from build123d import *

# Parameters (mm, degrees)
BASE_DEPTH                     = 3
CONG_1_R                       = 3
ESQUISSE20_R                   = 3
PER_AGE_PROFIL_S_DEPTH         = 4
ESQUISSE21_R                   = 1.65
PER_AGE_LIDAR_DEPTH            = 4
ESQUISSE22_R                   = 11.25
PER_AGE_ARRET_D_URGENCE_DEPTH  = 4
ESQUISSE23_R                   = 7
PER_AGE_TIRETTE_DEPTH          = 4
ESQUISSE24_W                   = 68
ESQUISSE24_H                   = 207
PER_AGE_CABLE_MANAGEMENT_DEPTH = 4


with BuildPart() as part:
    # Esquisse1 → Base (new body)
    with BuildSketch(Plane.XY):
        Polygon((0, 0), (-200, 0), (-224.748737342, 24.748737342), (-224.748737342, 284.748737342), (-200, 309.497474683), (0, 309.497474683), (24.748737342, 284.748737342), (24.748737342, 24.748737342), align=None)
    extrude(amount=BASE_DEPTH)

    # Congé1
    cong_1_edges = [part.edges().sort_by_distance(p)[0] for p in [
        (0, 0, 1.5),
        (-200, 0, 1.5),
        (-224.748737342, 24.748737342, 1.5),
        (-224.748737342, 284.748737342, 1.5),
        (-200, 309.497474683, 1.5),
        (0, 309.497474683, 1.5),
        (24.748737342, 284.748737342, 1.5),
        (24.748737342, 24.748737342, 1.5),
    ]]
    fillet(cong_1_edges, radius=CONG_1_R)

    # Esquisse20 → Perçage Profilés (cut, through all)
    with BuildSketch(Plane(origin=(0, 0, 0), x_dir=(-1, 0, 0), z_dir=(0, 0, -1))):
        with Locations((35, 286.497474683)):
            Circle(ESQUISSE20_R)
        with Locations((165, 286.497474683)):
            Circle(ESQUISSE20_R)
        with Locations((165, 23)):
            Circle(ESQUISSE20_R)
        with Locations((35, 23)):
            Circle(ESQUISSE20_R)
    extrude(amount=-PER_AGE_PROFIL_S_DEPTH, mode=Mode.SUBTRACT)

    # Esquisse21 → Perçage Lidar (cut, through all)
    with BuildSketch(Plane(origin=(0, 0, 0), x_dir=(-1, 0, 0), z_dir=(0, 0, -1))):
        with Locations((61, 154.748737342)):
            Circle(ESQUISSE21_R)
        with Locations((100, 115.748737342)):
            Circle(ESQUISSE21_R)
    extrude(amount=-PER_AGE_LIDAR_DEPTH, mode=Mode.SUBTRACT)

    # Esquisse22 → Perçage Arret d'urgence (cut, through all)
    with BuildSketch(Plane(origin=(0, 0, 0), x_dir=(-1, 0, 0), z_dir=(0, 0, -1))):
        with Locations((70, 65)):
            Circle(ESQUISSE22_R)
    extrude(amount=-PER_AGE_ARRET_D_URGENCE_DEPTH, mode=Mode.SUBTRACT)

    # Esquisse23 → Perçage Tirette (cut, through all)
    with BuildSketch(Plane(origin=(0, 0, 0), x_dir=(-1, 0, 0), z_dir=(0, 0, -1))):
        with Locations((130, 65)):
            Circle(ESQUISSE23_R)
    extrude(amount=-PER_AGE_TIRETTE_DEPTH, mode=Mode.SUBTRACT)

    # Esquisse24 → Perçage Cable management (cut, through all)
    with BuildSketch(Plane(origin=(0, 0, 0), x_dir=(-1, 0, 0), z_dir=(0, 0, -1))):
        with Locations((183.744364822, 157.241556094)):
            Rectangle(ESQUISSE24_W, ESQUISSE24_H)
    extrude(amount=-PER_AGE_CABLE_MANAGEMENT_DEPTH, mode=Mode.SUBTRACT)


solid = part.part
The listing builds one solid part. Answer for the finished solid, in the listing's coordinates (mm). Coordinates: 2 decimals unless noted, no trailing zeros. Order: outer loops, then holes, each group sorted by start corner. A loop starts at its lowest first (then second) coordinate and runs counter-clockwise, first axis right, second up. Notation, with made-up numbers: M 82,86 L 123,86 A15 ccw 123,93 Z; hole C 87,-33.75 d8. An arc over 180 degrees is marked long. Use CSV: the item, a comma, the result in double quotes.
Q1. Determine the mould class of faces 1 (the flat face through (-212, 12, 1)), 2 (the cylindrical face through (-32, 23, 1)), 3 (the flat face through (-71, 157, 3)) for opening direction X: pulls with the +X half, pulls with the -X half, needs draft (parallel to the pull), parting line crosses it, or undercut.
Here are the results:
face 1,"pulls with the -X half"
face 2,"undercut"
face 3,"needs draft"
Q2. Straight lines are drawn through the part: L1, parallel to Y at x = -35, z = 1.8; L2, parallel to X at y = 123.5, z = 2.2; L3, parallel to Y at x = -174.5, z = 0.85. For each, find the intervals that lie inside material, in ascending order.
Here are the results:
L1,"0 to 20, 26 to 283.5, 289.5 to 309.5"
L2,"-224.75 to -217.74, -149.74 to 24.75"
L3,"0 to 53.74, 260.74 to 309.5"
Q3. Given pin 1 Ø4 at (x, y) = (-61, 154.75) entering from -Z, flat-ended and moving along its own axis, determine where the tip first touches the part or whether it passes through.
Here are the results:
pin 1,"z = 0"
Q4. Section C-C (y = 65) is taken. Determine the outline of the cut face in (x, z), then the cut area to 3 significant figures.
Here are the results:
outline,"M -224.75,0 L -217.74,0 L -217.74,3 L -224.75,3 Z; M -149.74,0 L -137,0 L -137,3 L -149.74,3 Z; M -123,0 L -81.25,0 L -81.25,3 L -123,3 Z; M -58.75,0 L 24.75,0 L 24.75,3 L -58.75,3 Z"
area,"435 mm2"
Q5. Section B-B (y = 209.5) is taken. Determine the outline of the cut face in (x, z), then the cut area to 3 significant figures.
Here are the results:
outline,"M -224.75,0 L -217.74,0 L -217.74,3 L -224.75,3 Z; M -149.74,0 L 24.75,0 L 24.75,3 L -149.74,3 Z"
area,"544 mm2"
Q6. Section A-A (x = -130) is taken. Determine the outline of the cut face in (y, z), then the cut area to 3 significant figures.
Here are the results:
outline,"M 0,0 L 58,0 L 58,3 L 0,3 Z; M 72,0 L 309.5,0 L 309.5,3 L 72,3 Z"
area,"886 mm2"
Q7. Section D-D (z = 0.65) is taken. Give the number of separate pieces and of enclosed holes in the cut face, then the cut area to 3 significant figures.
Here are the results:
separate pieces,"1"
enclosed holes,"9"
area,"61,200 mm2"
